For this review, take the finished solid that the model builds, in its own axes (mm). Face numbers are marked on the shaded views. A direction names the side the tool comes from. Round coordinates to 2 decimals unless told otherwise and drop trailing zeros. Loops run counter-clockwise (first coordinate to the right, second up) from the corner with the lowest first, then second, coordinate; pieces in that order, holes last.
1) Tool access review of the marked faces 1, 2, 3 and 4: name each direction out of +Z, -Z, +X, -X, +Y, -Y from which nothing blocks a thin tool from reaching the whole face with its end or side.
2) Take a section at D-D (x = 2.25). State the section outline as (y, z) points, then the cut area to 3 significant figures.
3) Mouldability with a two-part tool opening along Z and no side actions: class the marked faces 5, 6 and 7 as pulls with the +Z half, pulls with the -Z half, needs draft (parallel to the pull), parting line crosses it, or undercut.
4) Take a section at C-C (z = 10). State the section outline as (x, y) points, then the cut area to 3 significant figures.
5) Take a section at A-A (x = 0). Give the number of separate pieces and of enclosed holes in the cut face, then the cut area to 3 significant figures.
6) Wall thickness on L1, parallel to Z at x = 0, y = 0.7; L2, parallel to X at y = 6.5, z = 10; L3, parallel to Y at x = 0, z = 2.3: over which ranges is each line inside the solid? List them lowest first.
7) Insertion check: pin 1 (2.5 mm diameter, centred on x = -1.5, z = 17, fed in from -Y); pin 2 (0.8 mm diameter, centred on x = 1.5, y = -0.5, fed in from +Z); pin 3 (1.9 mm diameter, centred on x = 0, z = -15.286, fed in from -Y); pin 4 (5 mm diameter, centred on x = -5, y = 17, fed in from -Z). Each pin has a flat end and moves straight along its axis. Give the tip position at first contact, or say it passes through.
8) Take a section at B-B (y = 25.9). State the section outline as (x, z) points, then the cut area to 3 significant figures.
```python
from build123d import *

# Parameters (mm, degrees)
SKETCH_R            = 4.1
PAD_DEPTH           = 6
SKETCH001_W         = 2.5
SKETCH001_H         = 14
PAD001_DEPTH        = 20
PAD002_DEPTH        = 14
PAD003_DEPTH        = 2
LINEARPATTERN_COUNT = 2
LINEARPATTERN_PITCH = 18
POCKET_DEPTH        = 20.001
PAD004_DEPTH        = 20
SKETCH004_R         = 1.6
POCKET001_DEPTH     = 34.561
SKETCH005_W         = 20
SKETCH005_H         = 2.5
PAD005_DEPTH        = 20
SKETCH006_W         = 20
SKETCH006_H         = 20
PAD006_DEPTH        = 3
SKETCH007_W         = 20
SKETCH007_H         = 20
PAD007_DEPTH        = 3
POCKET002_DEPTH     = 20.001
PAD008_DEPTH        = 19
SKETCH010_R         = 1.6
POCKET003_DEPTH     = 34.561


with BuildPart() as part:
    # Sketch → Pad (new body)
    with BuildSketch(Plane.XY):
        Polygon((-4.74, 0), (-2.94, -1.56), (2.94, -1.56), (4.74, 0), (10, 0), (10, 33), (-10, 33), (-10, 0), align=None)
        with Locations((0, 25.9)):
            Circle(SKETCH_R, mode=Mode.SUBTRACT)
    extrude(amount=PAD_DEPTH)

    # Sketch001 (on Face5 of Pad) → Pad001 (join)
    with BuildSketch(Plane.YZ.offset(10)):
        with Locations((1.25, 13)):
            Rectangle(SKETCH001_W, SKETCH001_H)
    extrude(amount=-PAD001_DEPTH)

    # Pad001 Face5 → Pad002 (add)
    with BuildSketch(Plane(origin=(0, -0.719062, 6), x_dir=(0, 1, 0), z_dir=(0, 0, 1))):
        Polygon((0.719062, -4.74), (0.719062, 4.74), (-0.840938, 2.94), (-0.840938, -2.94), align=None)
    extrude(amount=PAD002_DEPTH)

    # Sketch002 (on Face6 of Pad002) → Pad003 (join)
    with BuildSketch(Plane(origin=(-10, 0, 0), x_dir=(0, -1, 0), z_dir=(-1, 0, 0))):
        Polygon((-33, 6), (-2.5, 20), (-2.5, 6), align=None)
    pad003 = extrude(amount=-PAD003_DEPTH)

    # LinearPattern: Pad003 ×2
    with Locations(*[(i * LINEARPATTERN_PITCH, 0, 0) for i in range(1, LINEARPATTERN_COUNT)]):
        add(pad003)

    # LinearPattern Face14 → Pocket (cut, through all)
    with BuildSketch(Plane(origin=(0, -0.719062, 20), x_dir=(0, 1, 0), z_dir=(0, 0, 1))):
        Polygon((0.719062, -4.74), (0.719062, 4.74), (-0.840938, 2.94), (-0.840938, -2.94), align=None)
    extrude(amount=-POCKET_DEPTH, mode=Mode.SUBTRACT)

    # Sketch003 (on Face10 of Pocket) → Pad004 (join)
    with BuildSketch(Plane(origin=(-10, 0, 0), x_dir=(0, -1, 0), z_dir=(-1, 0, 0))):
        Polygon((0, 10), (0, 14.74), (1.56, 12.94), (1.56, 7.06), (0, 5.26), align=None)
    extrude(amount=-PAD004_DEPTH)

    # Sketch004 (on Face14 of Pad004) → Pocket001 (cut, through all)
    with BuildSketch(Plane.XZ.offset(1.56)):
        with Locations((0, 10)):
            Circle(SKETCH004_R)
    extrude(amount=-POCKET001_DEPTH, mode=Mode.SUBTRACT)

    # Sketch005 (on Face2 of Pocket001) → Pad005 (join)
    with BuildSketch(Plane(origin=(0, 0, 0), x_dir=(1, 0, 0), z_dir=(0, 0, -1))):
        with Locations((0, -1.25)):
            Rectangle(SKETCH005_W, SKETCH005_H)
    extrude(amount=PAD005_DEPTH)

    # Sketch006 (on Face18 of Pad005) → Pad006 (join)
    with BuildSketch(Plane.YZ.offset(10)):
        with Locations((12.5, -10)):
            Rectangle(SKETCH006_W, SKETCH006_H)
    extrude(amount=-PAD006_DEPTH)

    # Sketch007 (on Face3 of Pad006) → Pad007 (join)
    with BuildSketch(Plane(origin=(-10, 0, 0), x_dir=(0, -1, 0), z_dir=(-1, 0, 0))):
        with Locations((-12.5, -10)):
            Rectangle(SKETCH007_W, SKETCH007_H)
    extrude(amount=-PAD007_DEPTH)

    # Sketch008 (on Face18 of Pad007) → Pocket002 (cut, through all)
    with BuildSketch(Plane.YZ.offset(10)):
        Polygon((22.5, 0), (2.5, -20), (22.5, -20), align=None)
    extrude(amount=-POCKET002_DEPTH, mode=Mode.SUBTRACT)

    # Sketch009 (on Face9 of Pocket002) → Pad008 (join)
    with BuildSketch(Plane(origin=(0, 0, -20), x_dir=(1, 0, 0), z_dir=(0, 0, -1))):
        Polygon((0, 0), (-4.74, 0), (-2.94, 1.56), (2.94, 1.56), (4.74, 0), align=None)
    extrude(amount=-PAD008_DEPTH)

    # Sketch010 (on Face27 of Pad008) → Pocket003 (cut, through all)
    with BuildSketch(Plane.XZ.offset(1.56)):
        with Locations((0, -4.714)):
            Circle(SKETCH010_R)
        with Locations((0, -15.286)):
            Circle(SKETCH010_R)
    extrude(amount=-POCKET003_DEPTH, mode=Mode.SUBTRACT)


solid = part.part
```
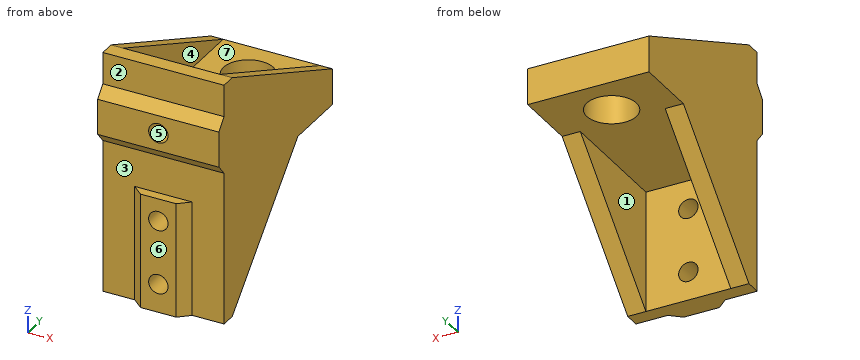
Response:
1. face 1: -Z, +Y
1. face 2: +Z, +X, -X, -Y
1. face 3: -Y
1. face 4: +Z, +Y
2. outline: (-1.56, -20) - (2.5, -20) - (2.5, 0) - (22.47, 0) - (22.47, 6) - (2.5, 6) - (2.5, 20) - (0, 20) - (0, 14.74) - (-1.56, 12.94) - (-1.56, 7.06) - (0, 5.26) - (0, -1) - (-1.56, -1) - close; (29.33, 0) - (33, 0) - (33, 6) - (29.33, 6) - close
2. area: 283 mm2
3. face 5: undercut
3. face 6: needs draft
3. face 7: pulls with the +Z half
4. outline: (-10, -1.56) - (-1.6, -1.56) - (-1.6, 2.5) - (-8, 2.5) - (-8, 24.29) - (-10, 24.29) - close; (1.6, -1.56) - (10, -1.56) - (10, 24.29) - (8, 24.29) - (8, 2.5) - (1.6, 2.5) - close
4. area: 155 mm2
5. separate pieces: 5
5. enclosed holes: 0
5. area: 236 mm2
6. L1: z = -20 to -16.89, -13.69 to -6.31, -3.11 to 8.4, 11.6 to 20
6. L2: x = -10 to -8, 8 to 10
6. L3: y = 0 to 21.8, 30 to 33
7. pin 1: stops at y = 0
7. pin 2: stops at z = 14.62
7. pin 3: passes through
7. pin 4: stops at z = -7
8. outline: (-10, 0) - (-4.1, 0) - (-4.1, 6) - (-8, 6) - (-8, 9.26) - (-10, 9.26) - close; (4.1, 0) - (10, 0) - (10, 9.26) - (8, 9.26) - (8, 6) - (4.1, 6) - close
8. area: 83.8 mm2
